Verification items for the finished model (mm, model axes). A direction names the side the tool comes from. Give positions to 0.01 mm unless a question says otherwise; leave off trailing zeros. Write each loop counter-clockwise with the first axis right and the second up, starting at its lowest first coordinate (ties: lowest second). Pieces come first, ordered by that corner, then holes. Notation, with made-up numbers: (-20, 69) -> (11, 69) arc R25 ccw to (11, 98) -> close; hole circle Ø9 at (82.25, 71). An arc over 180 degrees is marked (long way). Answer as CSV lines item,"result".
```python
from build123d import *

# Parameters (mm, degrees)
SKETCH_1_R      = 1.5
EXTRUDE_1_DEPTH = 3
FILLET_1_R      = 5


with BuildPart() as part:
    # 草图1 → 凸台-拉伸1 (new body)
    with BuildSketch(Plane.XY):
        Polygon((0, 0), (0, 65), (15, 65), (15, 15), (65, 15), (65, 0), align=None)
        with Locations((7.5, 57.5)):
            Circle(SKETCH_1_R, mode=Mode.SUBTRACT)
        with Locations((7.5, 37.5)):
            Circle(SKETCH_1_R, mode=Mode.SUBTRACT)
        with Locations((7.5, 17.5)):
            Circle(SKETCH_1_R, mode=Mode.SUBTRACT)
        with Locations(Location((57.5, 7.5, 0), (0, 0, 180))):
            Circle(SKETCH_1_R, mode=Mode.SUBTRACT)
        with Locations(Location((37.5, 7.5, 0), (0, 0, 180))):
            Circle(SKETCH_1_R, mode=Mode.SUBTRACT)
        with Locations(Location((17.5, 7.5, 0), (0, 0, 180))):
            Circle(SKETCH_1_R, mode=Mode.SUBTRACT)
    extrude(amount=EXTRUDE_1_DEPTH)

    # 圆角1
    fillet_1_edges = [part.edges().sort_by_distance(p)[0] for p in [
        (0, 0, 1.5),
        (0, 65, 1.5),
        (15, 65, 1.5),
        (65, 15, 1.5),
        (65, 0, 1.5),
    ]]
    fillet(fillet_1_edges, radius=FILLET_1_R)


solid = part.part
```
1) Section check D-D (z = 0.6). Record the boundary of the cut face in (x, y).
Reported:
outline,"(0, 5) arc R5 ccw to (5, 0) -> (60, 0) arc R5 ccw to (65, 5) -> (65, 10) arc R5 ccw to (60, 15) -> (15, 15) -> (15, 60) arc R5 ccw to (10, 65) -> (5, 65) arc R5 ccw to (0, 60) -> close; hole circle Ø3 at (7.5, 17.5); hole circle Ø3 at (7.5, 37.5); hole circle Ø3 at (7.5, 57.5); hole circle Ø3 at (17.5, 7.5); hole circle Ø3 at (37.5, 7.5); hole circle Ø3 at (57.5, 7.5)"
2) Draft check along X on faces 3 (the flat face through (33, 0, 1)), 4 (the cylindrical face through (1, 63, 2)), 5 (the cylindrical face through (56.114, 8.075, 1.479)). Enter one of: +X half, -X half, draft (parallel to the pull), parting line (faces both ways), or undercut.
Reported:
face 3,"draft"
face 4,"-X half"
face 5,"undercut"
3) Section check C-C (x = 37.5). Record the boundary of the cut face in (y, z).
Reported:
outline,"(0, 0) -> (6, 0) -> (6, 3) -> (0, 3) -> close; (9, 0) -> (15, 0) -> (15, 3) -> (9, 3) -> close"
4) Scan lines: line 1 along Y through (x, z) = (7.5, 1.4); line 2 along Y through (x, z) = (57.5, 1.55). Record each from-to range of solid material in increasing order.
Reported:
line 1,"0 to 16, 19 to 36, 39 to 56, 59 to 65"
line 2,"0 to 6, 9 to 15"
5) Tool access check on faces 1 (the flat face through (19, 11, 0)), 2 (the flat face through (37, 15, 1)). Record the directions out of +Z, -Z, +X, -X, +Y, -Y that give a thin tool (end or side, any length) a straight path to the whole face; none if there is none.
Reported:
face 1,"-Z, +X, -X, +Y, -Y"
face 2,"+Z, -Z, +X, +Y"
6) Section check A-A (x = 7.5). Record the boundary of the cut face in (y, z), and give its area (3 significant figures).
Reported:
outline,"(0, 0) -> (16, 0) -> (16, 3) -> (0, 3) -> close; (19, 0) -> (36, 0) -> (36, 3) -> (19, 3) -> close; (39, 0) -> (56, 0) -> (56, 3) -> (39, 3) -> close; (59, 0) -> (65, 0) -> (65, 3) -> (59, 3) -> close"
area,"168 mm²"
7) Depth check by flat-ended pin: pin 1 (2.5 mm diameter, centred on x = 7.5, y = 17.5, fed in from -Z); pin 2 (1.5 mm diameter, centred on y = 34.5, z = 1, fed in from +X); pin 3 (1.5 mm diameter, centred on x = 33.5, z = 2, fed in from +Y). Enter the tip coordinate at first touch or a pass-through.
Reported:
pin 1,"through"
pin 2,"x = 15"
pin 3,"y = 15"
